Check sheet for the modelled part. Datum: model origin and axes. Units: mm. Face numbers are marked on the shaded views. A direction names the side the tool comes from. Coordinates: 2 decimals unless noted, no trailing zeros. Write each loop counter-clockwise with the first axis right and the second up, starting at its lowest first coordinate (ties: lowest second). Pieces come first, ordered by that corner, then holes. Notation, with made-up numbers: (57, 61) - (73, 61) arc R26 cw to (73, 93) - close; hole circle Ø11 at (79.25, 84). An arc over 180 degrees is marked (long way). Write each question's results on one line, items separated by ' | '.
from build123d import *

# Parameters (mm, degrees)
EXTRUDE_1_DEPTH = 3
SKETCH_2_R      = 2.1
SKETCH_2_R_2    = 1.2
EXTRUDE_2_DEPTH = 3


with BuildPart() as part:
    # 草图1 → 凸台-拉伸1 (new body)
    with BuildSketch(Plane.XY):
        with BuildLine():
            Line((0.798434478, -20.883817003), (17.2756604, -12.326264758))
            ThreePointArc((17.2756604, -12.326264758), (17.48353375, -12.18227786), (17.648643158, -11.990751257))
            Line((17.648643158, -11.990751257), (24.128865743, -2.200202913))
            ThreePointArc((24.128865743, -2.200202913), (24.566982391, 0.053711846), (23.283019233, 1.957265509))
            Line((23.283019233, 1.957265509), (14.944161012, 7.476635362))
            ThreePointArc((14.944161012, 7.476635362), (14.192856092, 7.622674245), (13.558338205, 7.194686526))
            Line((13.558338205, 7.194686526), (11.902527249, 4.693029059))
            ThreePointArc((11.902527249, 4.693029059), (11.268009361, 4.26504134), (10.516704441, 4.411080223))
            Line((10.516704441, 4.411080223), (1.343960399, 10.482387061))
            ThreePointArc((1.343960399, 10.482387061), (0.915972679, 11.116904949), (1.062011562, 11.868209869))
            Line((1.062011562, 11.868209869), (2.717822518, 14.369867335))
            ThreePointArc((2.717822518, 14.369867335), (2.8638614, 15.121172254), (2.435873681, 15.755690142))
            Line((2.435873681, 15.755690142), (-5.069098717, 20.72312301))
            ThreePointArc((-5.069098717, 20.72312301), (-7.323013477, 21.161239658), (-9.22656714, 19.8772765))
            Line((-9.22656714, 19.8772765), (-24.128865743, -2.637640696))
            ThreePointArc((-24.128865743, -2.637640696), (-24.566982391, -4.891555455), (-23.283019233, -6.795109118))
            Line((-23.283019233, -6.795109118), (-2.240085668, -20.72312301))
            ThreePointArc((-2.240085668, -20.72312301), (-0.742710136, -21.217278992), (0.798434478, -20.883817003))
        make_face()
        with BuildLine():
            Line((3.65242583, -4.518851403), (1.415541705, -4.574406046))
            ThreePointArc((1.415541705, -4.574406046), (0.956150335, -4.699151193), (0.606483954, -5.022160797))
            ThreePointArc((0.606483954, -5.022160797), (0.479294259, -5.297811966), (0.44067804, -5.598925853))
            Line((0.44067804, -5.598925853), (0.520246584, -8.802719514))
            ThreePointArc((0.520246584, -8.802719514), (1.243652504, -9.738966959), (2.353824142, -9.329828428))
            Line((2.353824142, -9.329828428), (4.511139723, -6.070480125))
            ThreePointArc((4.511139723, -6.070480125), (4.55220049, -5.034323699), (3.65242583, -4.518851403))
        make_face(mode=Mode.SUBTRACT)
        with BuildLine():
            Line((-3.794049487, -4.70379003), (-9.955030272, -4.856802465))
            ThreePointArc((-9.955030272, -4.856802465), (-10.414421641, -4.981547612), (-10.764088023, -5.304557216))
            ThreePointArc((-10.764088023, -5.304557216), (-10.910126905, -6.055862136), (-10.482139186, -6.690380023))
            Line((-10.482139186, -6.690380023), (-4.214325339, -10.838955509))
            ThreePointArc((-4.214325339, -10.838955509), (-3.178168913, -10.880016276), (-2.662696618, -9.980241616))
            Line((-2.662696618, -9.980241616), (-2.76952968, -5.678653695))
            ThreePointArc((-2.76952968, -5.678653695), (-3.079888708, -4.979036863), (-3.794049487, -4.70379003))
        make_face(mode=Mode.SUBTRACT)
        with BuildLine():
            Line((1.346368171, -1.789163051), (9.413331456, -1.588814155))
            ThreePointArc((9.413331456, -1.588814155), (10.349578901, -0.865408235), (9.94044037, 0.244763403))
            Line((9.94044037, 0.244763403), (1.733593774, 5.676756668))
            ThreePointArc((1.733593774, 5.676756668), (0.982288854, 5.822795551), (0.347770967, 5.394807831))
            ThreePointArc((0.347770967, 5.394807831), (0.220581273, 5.119156662), (0.181965053, 4.818042775))
            Line((0.181965053, 4.818042775), (0.321848364, -0.814299386))
            ThreePointArc((0.321848364, -0.814299386), (0.632207392, -1.513916218), (1.346368171, -1.789163051))
        make_face(mode=Mode.SUBTRACT)
        with BuildLine():
            Line((-9.867573328, -2.067669438), (-3.863223021, -1.918547035))
            ThreePointArc((-3.863223021, -1.918547035), (-3.163606189, -1.608188007), (-2.888359356, -0.894027228))
            Line((-2.888359356, -0.894027228), (-3.10194101, 7.705747447))
            ThreePointArc((-3.10194101, 7.705747447), (-3.82534693, 8.641994892), (-4.935518568, 8.232856362))
            Line((-4.935518568, 8.232856362), (-10.726287221, -0.516040717))
            ThreePointArc((-10.726287221, -0.516040717), (-10.767347988, -1.552197143), (-9.867573328, -2.067669438))
        make_face(mode=Mode.SUBTRACT)
        with BuildLine():
            ThreePointArc((17.521345347, -0.225190454), (17.972463486, -2.442506946), (20.189779977, -1.991388807))
            ThreePointArc((20.189779977, -1.991388807), (19.738661839, 0.225927685), (17.521345347, -0.225190454))
        make_face(mode=Mode.SUBTRACT)
        with BuildLine():
            ThreePointArc((-3.64705761, -14.995048823), (-3.054965053, -17.905276719), (-0.144737158, -17.313184161))
            ThreePointArc((-0.144737158, -17.313184161), (-0.736829715, -14.402956266), (-3.64705761, -14.995048823))
        make_face(mode=Mode.SUBTRACT)
        with BuildLine():
            ThreePointArc((-20.324774052, -3.956309117), (-19.732681494, -6.866537012), (-16.822453599, -6.274444455))
            ThreePointArc((-16.822453599, -6.274444455), (-17.414546156, -3.36421656), (-20.324774052, -3.956309117))
        make_face(mode=Mode.SUBTRACT)
        with BuildLine():
            ThreePointArc((-7.495229315, 16.332919105), (-7.044111176, 14.115602614), (-4.826794685, 14.566720752))
            ThreePointArc((-4.826794685, 14.566720752), (-5.277912823, 16.784037244), (-7.495229315, 16.332919105))
        make_face(mode=Mode.SUBTRACT)
    extrude(amount=EXTRUDE_1_DEPTH)

    # 草图2 → 凸台-拉伸2 (add)
    # profile 1 of 2: a face of its own
    with BuildSketch(Plane(origin=(0, 0, 0), x_dir=(-1, 0, 0), z_dir=(0, 0, -1))):
        with Locations((1.895897384, -16.154116492)):
            Circle(SKETCH_2_R)
        with Locations((1.895897384, -16.154116492)):
            Circle(SKETCH_2_R_2, mode=Mode.SUBTRACT)
    # profile 2 of 2: a face of its own
    with BuildSketch(Plane(origin=(0, 0, 0), x_dir=(-1, 0, 0), z_dir=(0, 0, -1))):
        with Locations((18.573613825, -5.115376786)):
            Circle(SKETCH_2_R)
        with Locations((18.573613825, -5.115376786)):
            Circle(SKETCH_2_R_2, mode=Mode.SUBTRACT)
    extrude(amount=-EXTRUDE_2_DEPTH)


solid = part.part
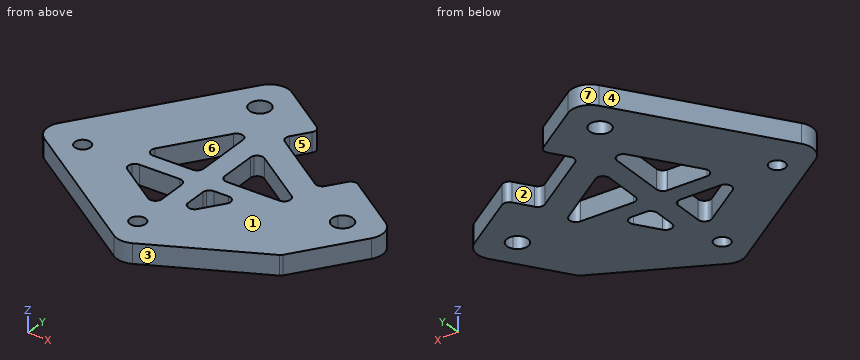
1. Access from +Z, -Z, +X, -X, +Y, -Y to the whole of each face (thin tool, end or side, straight path). Record for the marked faces 5, 6 and 7.
Values follow:
face 5: +Z, -Z, +X | face 6: +Z, -Z | face 7: +Z, -Z, +Y
2. Go/stop test with flat-tipped pins: pin 1 (2.5 mm diameter, centred on x = -6.16, y = 15.45, fed in from -Z); pin 2 (1 mm diameter, centred on y = 11, z = 2, fed in from +X). Record where each tip stops, or that it passes through.
Values follow:
pin 1: passes through | pin 2: stops at x = 1.32
3. Sectioned sample at A-A (x = 7). Record the cut outline in (y, z), then the cut area to 3 significant figures.
Values follow:
outline: (-17.66, 0) - (-1.65, 0) - (-1.65, 3) - (-17.66, 3) - close; (2.19, 0) - (6.74, 0) - (6.74, 3) - (2.19, 3) - close | area: 61.7 mm^2
4. Draft check along X on the marked faces 1, 2, 3 and 4. Enter one of: pulls with the +X half, pulls with the -X half, needs draft (parallel to the pull), parting line crosses it, or undercut.
Values follow:
face 1: needs draft | face 2: undercut | face 3: pulls with the +X half | face 4: pulls with the -X half
5. Sectioned sample at B-B (x = -7). Record the cut outline in (y, z), then the cut area to 3 significant figures.
Values follow:
outline: (-17.57, 0) - (-9, 0) - (-9, 3) - (-17.57, 3) - close; (-4.78, 0) - (-2, 0) - (-2, 3) - (-4.78, 3) - close; (5.11, 0) - (14.09, 0) - (14.09, 3) - (5.11, 3) - close; (16.81, 0) - (21.21, 0) - (21.21, 3) - (16.81, 3) - close | area: 74.2 mm^2
6. Material ranges on L1, parallel to X at y = 7, z = 1.15; L2, parallel to Y at x = -10, z = 1.65; L3, parallel to Y at x = -3.5, z = 2.75, recorded low to high. Write a range as [from, to].
Values follow:
L1: x = [-17.75, -5.75], [-3.08, 6.61], [13.43, 15.66] | L2: y = [-15.59, -7.01], [-4.86, -2.06], [0.58, 18.71] | L3: y = [-19.89, -10.99], [-4.74, -1.84], [8.48, 19.68]
7. Sectioned sample at C-C (z = 2.55). Give the number of separate pieces and of enclosed holes in the cut face, then the cut area to 3 significant figures.
Values follow:
separate pieces: 1 | enclosed holes: 8 | area: 980 mm^2
8. Sectioned sample at D-D (y = 18.5). Record the cut outline in (x, z).
Values follow:
outline: (-10.14, 0) - (-1.71, 0) - (-1.71, 3) - (-10.14, 3) - close
